from build123d import *

# Parameters (mm, degrees)
SKETCH_1_W          = 28
SKETCH_1_H          = 10.3
EXTRUDE_1_DEPTH     = 16
SKETCH_2_R          = 1.6
CUT_EXTRUDE_1_DEPTH = 16
FILLET_1_R          = 3
EXTRUDE_START       = -3.05
EXTRUDE_2_DEPTH     = 4.2
SKETCH_4_W          = 5
SKETCH_4_H          = 0.5
EXTRUDE_3_DEPTH     = 10.3
SKETCH_5_W          = 6.8
SKETCH_5_H          = 0.1
CUT_EXTRUDE_2_DEPTH = 12.2
EXTRUDE_START_2     = -2
EXTRUDE_4_DEPTH     = 6.3


with BuildPart() as part:
    # 草图1 → 凸台-拉伸1 (new body)
    with BuildSketch(Plane(origin=(0, 0, 0), x_dir=(1, 0, 0), z_dir=(0, 1, 0))):
        with Locations((14, 5.15)):
            Rectangle(SKETCH_1_W, SKETCH_1_H)
    extrude(amount=EXTRUDE_1_DEPTH)

    # 草图2 → 切除-拉伸1 (cut)
    with BuildSketch(Plane.XY):
        with Locations((2.9, 2.9)):
            Circle(SKETCH_2_R)
        with Locations((25.1, 13.1)):
            Circle(SKETCH_2_R)
    extrude(amount=-CUT_EXTRUDE_1_DEPTH, mode=Mode.SUBTRACT)

    # 圆角1
    fillet_1_edges = [part.edges().sort_by_distance(p)[0] for p in [
        (28, 16, -5.15),
        (0, 16, -5.15),
        (28, 0, -5.15),
        (0, 0, -5.15),
    ]]
    fillet(fillet_1_edges, radius=FILLET_1_R)

    # 草图3 → 凸台-拉伸2 (add)
    with BuildSketch(Plane.XY.offset(EXTRUDE_START)):
        with BuildLine():
            Line((3.8, 16), (3.8, 17.7))
            ThreePointArc((3.8, 17.7), (4.8, 18.7), (5.8, 17.7))
            Line((5.8, 17.7), (5.8, 16))
            Line((5.8, 16), (3.8, 16))
        make_face()
    extrude(amount=-EXTRUDE_2_DEPTH)

    # 草图4 → 凸台-拉伸3 (add)
    with BuildSketch(Plane(origin=(28, 0, 0), x_dir=(0, 0, -1), z_dir=(1, 0, 0))):
        with Locations((5.15, 10.95)):
            Rectangle(SKETCH_4_W, SKETCH_4_H)
        with Locations((5.15, 5.05)):
            Rectangle(SKETCH_4_W, SKETCH_4_H)
    extrude(amount=EXTRUDE_3_DEPTH)

    # 草图5 → 切除-拉伸2 (cut, through all)
    with BuildSketch(Plane(origin=(0, 11.2, 0), x_dir=(1, 0, 0), z_dir=(0, 1, 0))):
        with Locations((34.9, 7.6)):
            Rectangle(SKETCH_5_W, SKETCH_5_H)
        with Locations((34.9, 2.7)):
            Rectangle(SKETCH_5_W, SKETCH_5_H)
    extrude(amount=-CUT_EXTRUDE_2_DEPTH, mode=Mode.SUBTRACT)

    # 草图6 → 凸台-拉伸4 (add)
    with BuildSketch(Plane.XY.offset(EXTRUDE_START_2)):
        Polygon((14, 0), (14, -3.2), (25, -3.2), (25, -2.2), (15, -2.2), (15, 0), align=None)
    extrude(amount=-EXTRUDE_4_DEPTH)


solid = part.part
Build history of the part. All positions in model axes, mm. A direction names the side the tool comes from. Coordinates: 2 decimals unless noted, no trailing zeros. Order: outer loops, then holes, each group sorted by start corner. A loop starts at its lowest first (then second) coordinate and runs counter-clockwise, first axis right, second up. Notation, with made-up numbers: (82, 86) - (132, 86) arc R29 ccw to (132, 109) - close; hole circle Ø7 at (-24.75, 4). An arc over 180 degrees is marked (long way). Write each question's results on one line, items separated by ' | '. Start each with the question number.
Item 1: Band-saw the part on D-D on z = -0.5. Write the cut outline in (x, y), and give its area (3 significant figures).
Item 2: Flat gauge pins, fed straight in: pin 1 (0.6 mm diameter, centred on x = 4.5, y = 18, fed in from -Z); pin 2 (2.5 mm diameter, centred on x = 32.5, z = -5, fed in from +Y); pin 3 (0.5 mm diameter, centred on y = 16.5, z = -4.5, fed in from -X). Where does each tip first touch, or does it go through?
Item 3: Tool access for faces 4 (the face through (18, -3, -8.3)), 5 (the face through (3.8, 17, -5)), 6 (the face through (15, -1, -5)), 7 (the face through (18, -3, -2)), 8 (the face through (5, 17, -7.25)): list every direction of +Z, -Z, +X, -X, +Y, -Y with a clear straight run to the whole face (end or side of a thin tool).
Item 4: Wall check: probe 1 along Y at (x, z) = (2.9, -6); probe 2 along Y at (x, z) = (25.1, -2.5); probe 3 along X at (y, z) = (2.75, -3.5). Give the ranges that are in metal, low to high. Write a range as [from, to].
Item 5: Band-saw the part on C-C on y = 3.5. Write the cut outline in (x, z).
Item 6: Mould opens along Y. For faces 1 (the face through (23.92, 14.18, -5.08)), 2 (the face through (14, 8, 0)), 3 (the face through (0.86, 0.9, -5.22)) say: released by +Y, released by -Y, zero draft, split by the parting line, or undercut.
Item 7: Band-saw the part on A-A on z = -5. Write the cut outline in (x, y), and give its area (3 significant figures).
Item 8: Band-saw the part on B-B on x = 25.5. Write the cut outline in (y, z), and give its area (3 significant figures).
Numbers:
1) outline: (0, 3) arc R3 ccw to (3, 0) - (25, 0) arc R3 ccw to (28, 3) - (28, 13) arc R3 ccw to (25, 16) - (3, 16) arc R3 ccw to (0, 13) - close; hole circle Ø3.2 at (2.9, 2.9); hole circle Ø3.2 at (25.1, 13.1) | area: 424 mm^2
2) pin 1: z = -7.25 | pin 2: y = 11.2 | pin 3: x = 3.8
3) face 4: -Z, +X, -X, -Y | face 5: +Z, -Z, -X, +Y | face 6: +Z, -Z, +X | face 7: +Z, +X, -X, -Y | face 8: -Z, +X, -X, +Y
4) probe 1: [0, 1.3], [4.5, 16] | probe 2: [0, 11.5], [14.7, 16] | probe 3: [0.01, 1.31], [4.49, 27.99]
5) outline: (0, -10.3) - (1.42, -10.3) - (1.42, 0) - (0, 0) - close; (4.38, -10.3) - (28, -10.3) - (28, 0) - (4.38, 0) - close
6) face 1: undercut | face 2: zero draft | face 3: released by -Y
7) outline: (0, 3) arc R3 ccw to (3, 0) - (14, 0) - (14, -3.2) - (25, -3.2) - (25, -2.2) - (15, -2.2) - (15, 0) - (25, 0) arc R3 ccw to (28, 3) - (28, 4.8) - (38.3, 4.8) - (38.3, 5.3) - (28, 5.3) - (28, 10.7) - (38.3, 10.7) - (38.3, 11.2) - (28, 11.2) - (28, 13) arc R3 ccw to (25, 16) - (5.8, 16) - (5.8, 17.7) arc R1 ccw to (3.8, 17.7) - (3.8, 16) - (3, 16) arc R3 ccw to (0, 13) - close; hole circle Ø3.2 at (2.9, 2.9); hole circle Ø3.2 at (25.1, 13.1) | area: 453 mm^2
8) outline: (0.04, -10.3) - (11.55, -10.3) - (11.55, 0) - (0.04, 0) - close; (14.65, -10.3) - (15.96, -10.3) - (15.96, 0) - (14.65, 0) - close | area: 132 mm^2
